```python
from build123d import *

# Parameters (mm, degrees)
F2_DEPTH = 3
F3_ANGLE = -180


with BuildPart() as f2:
    # F1 (on Top) → F2 (new body)
    with BuildSketch(Plane.XY):
        with BuildLine():
            ThreePointArc((9.5394564345, 61.4916072786), (7.7716894816, 60.7593742316), (7.0394564345, 58.9916072786))
            Line((7.0394564345, 58.9916072786), (7.0394564345, -17.6715264808))
            ThreePointArc((7.0394564345, -17.6715264808), (7.7716894816, -19.4392934337), (9.5394564345, -20.1715264808))
            Line((9.5394564345, -20.1715264808), (61.973710984, -20.1715264808))
            ThreePointArc((61.973710984, -20.1715264808), (63.741477937, -19.4392934337), (64.473710984, -17.6715264808))
            Line((64.473710984, -17.6715264808), (64.473710984, 58.9916072786))
            ThreePointArc((64.473710984, 58.9916072786), (63.741477937, 60.7593742316), (61.973710984, 61.4916072786))
            Line((61.973710984, 61.4916072786), (9.5394564345, 61.4916072786))
        make_face()
        with BuildLine():
            ThreePointArc((10.0394564345, 29.5111155982), (10.339726047, 30.6990491915), (11.1684054122, 31.6016224971))
            Line((11.1684054122, 31.6016224971), (14.3762351945, 33.7054654956))
            ThreePointArc((14.3762351945, 33.7054654956), (14.9139294436, 33.9719729133), (15.4996438847, 34.1026630155))
            Line((15.4996438847, 34.1026630155), (41.488379603, 36.6897513669))
            ThreePointArc((41.488379603, 36.6897513669), (42.9909448679, 36.3642607287), (44.0189190549, 35.2210566343))
            Line((44.0189190549, 35.2210566343), (49.7887253608, 22.2949045332))
            ThreePointArc((49.7887253608, 22.2949045332), (49.8705715629, 20.4647296223), (48.6825547612, 19.0701490101))
            Line((48.6825547612, 19.0701490101), (38.8881494106, 13.8450064155))
            ThreePointArc((38.8881494106, 13.8450064155), (38.0588591774, 13.5750123576), (37.187286277, 13.6063135007))
            Line((37.187286277, 13.6063135007), (12.0153198212, 19.0036871275))
            ThreePointArc((12.0153198212, 19.0036871275), (10.5951903091, 19.8765568437), (10.0394564345, 21.4481258791))
            Line((10.0394564345, 21.4481258791), (10.0394564345, 29.5111155982))
        make_face(mode=Mode.SUBTRACT)
        with BuildLine():
            ThreePointArc((15.9272251247, 58.4916072786), (17.8426196837, 57.5982384383), (18.38909119, 55.5566182253))
            Line((18.38909119, 55.5566182253), (15.2479060665, 37.7787523161))
            ThreePointArc((15.2479060665, 37.7787523161), (14.3926711609, 36.2983468103), (12.7860400011, 35.7137413693))
            Line((12.7860400011, 35.7137413693), (11.5394564345, 35.7137413693))
            ThreePointArc((11.5394564345, 35.7137413693), (10.4787962628, 36.1530811975), (10.0394564345, 37.2137413693))
            Line((10.0394564345, 37.2137413693), (10.0394564345, 55.9916072786))
            ThreePointArc((10.0394564345, 55.9916072786), (10.7716894816, 57.7593742316), (12.5394564345, 58.4916072786))
            Line((12.5394564345, 58.4916072786), (15.9272251247, 58.4916072786))
        make_face(mode=Mode.SUBTRACT)
        with BuildLine():
            Line((42.1746714548, 39.6185510587), (20.7860221636, 37.4893853296))
            ThreePointArc((20.7860221636, 37.4893853296), (18.6852371117, 38.299036692), (18.0873754635, 40.4696114113))
            Line((18.0873754635, 40.4696114113), (21.3054426802, 56.4841289415))
            ThreePointArc((21.3054426802, 56.4841289415), (22.1723549039, 57.9256838227), (23.7564470481, 58.4916072786))
            Line((23.7564470481, 58.4916072786), (37.8007872021, 58.4916072786))
            ThreePointArc((37.8007872021, 58.4916072786), (38.7453269087, 58.3063091477), (39.5498494615, 57.7778830727))
            Line((39.5498494615, 57.7778830727), (49.7784843846, 47.7623415937))
            ThreePointArc((49.7784843846, 47.7623415937), (50.5156898059, 45.7143923011), (49.3682772196, 43.8647943731))
            Line((49.3682772196, 43.8647943731), (43.265884217, 39.994984051))
            ThreePointArc((43.265884217, 39.994984051), (42.7423014517, 39.7429249823), (42.1746714548, 39.6185510587))
        make_face(mode=Mode.SUBTRACT)
        with BuildLine():
            ThreePointArc((46.0133442347, 36.2574461736), (45.9085359015, 38.0173085241), (46.991124046, 39.4087477749))
            Line((46.991124046, 39.4087477749), (51.6493053984, 42.2598926234))
            ThreePointArc((51.6493053984, 42.2598926234), (53.0758807488, 42.6246485541), (54.4603215443, 42.1231629578))
            Line((54.4603215443, 42.1231629578), (60.4469597614, 37.6055030683))
            ThreePointArc((60.4469597614, 37.6055030683), (61.1709104619, 36.7403261682), (61.4408153873, 35.6449782708))
            Line((61.4408153873, 35.6449782708), (61.4734654473, 33.3155527949))
            ThreePointArc((61.4734654473, 33.3155527949), (61.4736495991, 33.2980344991), (61.473710984, 33.2805153429))
            Line((61.473710984, 33.2805153429), (61.473710984, 21.7292172013))
            ThreePointArc((61.473710984, 21.7292172013), (60.5127092735, 19.7590689163), (58.3685235721, 19.3035733287))
            Line((58.3685235721, 19.3035733287), (54.162405597, 20.35298115))
            ThreePointArc((54.162405597, 20.35298115), (53.161382251, 20.8628779095), (52.4846958892, 21.7596153363))
            Line((52.4846958892, 21.7596153363), (46.0133442347, 36.2574461736))
        make_face(mode=Mode.SUBTRACT)
        with BuildLine():
            Line((57.524509199, 42.3068744408), (55.8126571334, 43.9830634434))
            ThreePointArc((55.8126571334, 43.9830634434), (55.1067308347, 45.2970774673), (55.2747666339, 46.7792140212))
            Line((55.2747666339, 46.7792140212), (56.6867582251, 49.9767966496))
            ThreePointArc((56.6867582251, 49.9767966496), (59.4897623878, 51.4130802722), (61.473710984, 48.9669218659))
            Line((61.473710984, 48.9669218659), (61.473710984, 44.5015785165))
            ThreePointArc((61.473710984, 44.5015785165), (61.2884128531, 43.5570388099), (60.7599867781, 42.7525162571))
            Line((60.7599867781, 42.7525162571), (60.3527796418, 42.3366452686))
            ThreePointArc((60.3527796418, 42.3366452686), (58.9448101607, 41.736005867), (57.524509199, 42.3068744408))
        make_face(mode=Mode.SUBTRACT)
        with BuildLine():
            Line((51.0285760641, 50.1903671406), (45.7683108872, 55.3410450625))
            ThreePointArc((45.7683108872, 55.3410450625), (45.2002064135, 58.0657974579), (47.504283237, 59.6272865873))
            Line((47.504283237, 59.6272865873), (57.2054807654, 59.6780824029))
            ThreePointArc((57.2054807654, 59.6780824029), (58.1570472763, 59.4952834054), (58.9676329344, 58.9643924665))
            Line((58.9676329344, 58.9643924665), (59.3005865812, 58.6383752525))
            ThreePointArc((59.3005865812, 58.6383752525), (60.0513858333, 56.8784134011), (59.337800116, 55.1030371989))
            Line((59.337800116, 55.1030371989), (54.5639141177, 50.2275806753))
            ThreePointArc((54.5639141177, 50.2275806753), (52.8039522663, 49.4767814233), (51.0285760641, 50.1903671406))
        make_face(mode=Mode.SUBTRACT)
    extrude(amount=F2_DEPTH)


with BuildPart() as f3_1:
    # F3: copy of F2
    add(f2.part.rotate(Axis((35.7565837093, -20.1715264808, 3), (1, 0, 0)), F3_ANGLE))


solid = f2.part
```
Can you work these out from the model? Positions are in its coordinate system, mm. A direction names the side the tool comes from. Give positions to 0.01 mm unless a question says otherwise; leave off trailing zeros. Order: outer loops, then holes, each group sorted by start corner. A loop starts at its lowest first (then second) coordinate and runs counter-clockwise, first axis right, second up. Notation, with made-up numbers: M 5,-28 L 32,-28 A32 cw 32,8 Z; hole C 36.5,-36 d7. An arc over 180 degrees is marked long. One line per item, written item: value.
1) I want a section at B-B, the plane z = 0.7. Count the separate pieces of the cut face and the enclosed holes in it, plus the area to 3 significant figures.
Answer sheet:
separate pieces: 1
enclosed holes: 6
area: 2,900 mm^2
2) For P1, Ø12, axis at x = 54.5, y = 7.5, coming from the -Z side, with a flat end and sliding along its axis, tell me the tip position at first contact or that it passes through.
Answer sheet:
P1: stops at z = 0
3) On a 3-axis mill with a long thin cutter (end or side, diameter ignored), from which of +Z, -Z, +X, -X, +Y, -Y can I reach the whole of each face in a straight line? I mean faces 1 (the face through (28.312, 35.378, 1.479)), 2 (the face through (63.8, 60.7, 1.5)). Say none if no direction works.
Answer sheet:
face 1: +Z, -Z
face 2: +Z, -Z, +X, +Y
4) I want a section at A-A, the plane x = 31.5. List the corners of the cut face in (y, z) for me, plus the area to 3 significant figures.
Answer sheet:
outline: M -20.17,0 L 14.83,0 L 14.83,3 L -20.17,3 Z; M 35.7,0 L 38.56,0 L 38.56,3 L 35.7,3 Z; M 58.49,0 L 61.49,0 L 61.49,3 L 58.49,3 Z
area: 123 mm^2
5) Please list where these lines run through material, in increasing order: line 1 along Y through (x, z) = (58, 1.95); line 2 along X through (y, z) = (50, 1.2); line 3 along Y through (x, z) = (31.5, 1.8).
Answer sheet:
line 1: y = -20.17 to 19.4, 39.45 to 41.96, 51.27 to 53.74, 59.55 to 61.49
line 2: x = 7.04 to 10.04, 17.41 to 20, 47.49 to 51.25, 54.31 to 56.7, 61.25 to 64.47
line 3: y = -20.17 to 14.83, 35.7 to 38.56, 58.49 to 61.49
6) We'd pull the mould along Y, two halves only. Please class faces 3 (the face through (14.411, 36.314, 1.479)), 4 (the face through (36, 61.492, 1)), 5 (the face through (63.72, -19.46, 1.48)): released by +Y, released by -Y, zero draft, split by the parting line, or undercut.
Answer sheet:
face 3: undercut
face 4: released by +Y
face 5: released by -Y
